from build123d import *

# Parameters (mm, degrees)
F0_W     = 20
F0_H     = 20
F1_DEPTH = 2
F2_W     = 20
F2_H     = 20
F3_DEPTH = 25
F5_W     = 9
F5_H     = 9
F6_DEPTH = 7
F7_R     = 1
F8_DEPTH = 18
F9_DEPTH = 24.8
F10_R    = 0.8
F11_R    = 0.8


with BuildPart() as f1:
    # F0 (on Top) → F1 (new body)
    with BuildSketch(Plane.XY):
        Rectangle(F0_W, F0_H)
    extrude(amount=F1_DEPTH)

    # F2 (on face) → F3 (join)
    with BuildSketch(Plane.XY.offset(2)):
        Rectangle(F2_W, F2_H)
        Polygon((0, -4.5), (-4.5, -4.5), (-4.5, 0), (-4.5, 4.5), (0, 4.5), (4.5, 4.5), (4.5, 0), (4.5, -4.5), align=None, mode=Mode.SUBTRACT)
    extrude(amount=F3_DEPTH)

    # F5 (on face) → F6 (cut)
    with BuildSketch(Plane.XY.offset(27)):
        Polygon((3.7816442632, -6.55), (7.5632885264, 0), (3.7816442632, 6.55), (-3.7816442632, 6.55), (-7.5632885264, 0), (-3.7816442632, -6.55), align=None)
        Rectangle(F5_W, F5_H, mode=Mode.SUBTRACT)
    extrude(amount=-F6_DEPTH, mode=Mode.SUBTRACT)

    # F7
    f7_edges = [f1.edges().sort_by_distance(p)[0] for p in [
        (3.781644, -6.55, 23.5),
        (7.563289, 0, 23.5),
        (3.781644, 6.55, 23.5),
        (-3.781644, 6.55, 23.5),
        (-7.563289, 0, 23.5),
        (-3.781644, -6.55, 23.5),
    ]]
    fillet(f7_edges, radius=F7_R)

    # F2 (on face) → F8 (join)
    with BuildSketch(Plane.XY.offset(2)):
        Rectangle(F2_W, F2_H)
        Polygon((0, -4.5), (-4.5, -4.5), (-4.5, 0), (-4.5, 4.5), (0, 4.5), (4.5, 4.5), (4.5, 0), (4.5, -4.5), align=None, mode=Mode.SUBTRACT)
        with BuildLine():
            ThreePointArc((4.5, 0), (3.1819805153, -3.1819805153), (0, -4.5))
            Line((0, -4.5), (4.5, -4.5))
            Line((4.5, -4.5), (4.5, 0))
        make_face()
        with BuildLine():
            Line((-4.5, 0), (-4.5, -4.5))
            Line((-4.5, -4.5), (0, -4.5))
            ThreePointArc((0, -4.5), (-3.1819805153, -3.1819805153), (-4.5, 0))
        make_face()
        with BuildLine():
            Line((-4.5, 4.5), (-4.5, 0))
            ThreePointArc((-4.5, 0), (-3.1819805153, 3.1819805153), (0, 4.5))
            Line((0, 4.5), (-4.5, 4.5))
        make_face()
        with BuildLine():
            ThreePointArc((0, 4.5), (3.1819805153, 3.1819805153), (4.5, 0))
            Line((4.5, 0), (4.5, 4.5))
            Line((4.5, 4.5), (0, 4.5))
        make_face()
    extrude(amount=F8_DEPTH)

    # F4 (on face) → F9 (cut, symmetric)
    with BuildSketch(Plane.XZ.offset(10)):
        with BuildLine():
            Line((-4.0082180343, 0), (4.0082180343, 0))
            ThreePointArc((4.0082180343, 0), (0, 4.0082180343), (-4.0082180343, 0))
        make_face()
    extrude(amount=F9_DEPTH, both=True, mode=Mode.SUBTRACT)

    # F10
    f10_edges = [f1.edges().sort_by_distance(p)[0] for p in [
        (4.008218, 0, 0),
        (-4.008218, 0, 0),
    ]]
    fillet(f10_edges, radius=F10_R)

    # F11
    f11_edges = [f1.edges().sort_by_distance(p)[0] for p in [
        (10, -10, 13.5),
        (-10, -10, 13.5),
        (-10, 10, 13.5),
        (10, 10, 13.5),
    ]]
    fillet(f11_edges, radius=F11_R)


solid = f1.part
Can you work these out from the model? Positions are in its coordinate system, mm. A direction names the side the tool comes from. Coordinates: 2 decimals unless noted, no trailing zeros. Write each loop counter-clockwise with the first axis right and the second up, starting at its lowest first coordinate (ties: lowest second). Pieces come first, ordered by that corner, then holes. Notation, with made-up numbers: (42.5, -24.75) - (51.5, -24.75) arc R13 cw to (51.5, -10.75) - close; hole circle Ø10 at (-27.5, -18.5). An arc over 180 degrees is marked (long way). Return JSON: item names as keys, results as strings. Group by question number.
Item 1: If we section it at C-C (y = 8.25): Write out the boundary of the cut face in (x, z), then the cut area to 3 significant figures.
Item 2: If we section it at A-A (z = 13): Write out the boundary of the cut face in (x, y), then the cut area to 3 significant figures.
Item 3: We'd pull the mould along X, two halves only. Please class faces 3 (the face through (4, 0, 2)), 4 (the face through (0, 7, 27)), 5 (the face through (10, 0, 13)): pulls with the +X half, pulls with the -X half, needs draft (parallel to the pull), parting line crosses it, or undercut.
Item 4: Which directions (+Z, -Z, +X, -X, +Y, -Y) give clear straight access to the entire face, cutting with the end or side of a thin tool? Please do faces 1 (the face through (9.76, 9.77, 13.31)), 2 (the face through (7.41, -0.01, 23.45)).
Item 5: If we section it at B-B (x = 1): Write out the boundary of the cut face in (y, z).
Item 6: If we section it at D-D (y = -4): Write out the boundary of the cut face in (x, z), then the cut area to 3 significant figures.
Item 7: Please list where these lines run through material, in increasing order: probe 1 along X at (y, z) = (-2, 15.5); probe 2 along X at (y, z) = (-1, 9); probe 3 along Y at (x, z) = (4, 20.75).
Item 8: I'm going to push flat-ended pins straight in: pin 1 Ø3 at (x, y) = (1.5, 0) entering from +Z; pin 2 Ø8 at (x, y) = (-2, 6.5) entering from -Z; pin 3 Ø4 at (x, y) = (3, -1) entering from +Z. Where does each tip first touch, or does it pass through?
Return value:
{
 "1": {"outline": "(-10, 0) - (-4.74, 0) arc R0.8 ccw to (-3.95, 0.67) arc R4.01 cw to (3.95, 0.67) arc R0.8 ccw to (4.74, 0) - (10, 0) - (10, 27) - (-10, 27) - close", "area": "515 mm^2"},
 "2": {"outline": "(-10, -9.2) arc R0.8 ccw to (-9.2, -10) - (9.2, -10) arc R0.8 ccw to (10, -9.2) - (10, 9.2) arc R0.8 ccw to (9.2, 10) - (-9.2, 10) arc R0.8 ccw to (-10, 9.2) - close; hole circle Ø9 at (0, 0)", "area": "336 mm^2"},
 "3": {"face 3": "undercut", "face 4": "needs draft", "face 5": "pulls with the +X half"},
 "4": {"face 1": "+Z, -Z, +X, +Y", "face 2": "+Z"},
 "5": {"outline": "(-10, 3.88) - (-4.39, 3.88) - (-4.39, 20) - (-6.55, 20) - (-6.55, 27) - (-10, 27) - close; (4.39, 3.88) - (10, 3.88) - (10, 27) - (6.55, 27) - (6.55, 20) - (4.39, 20) - close"},
 "6": {"outline": "(-10, 0) - (-4.74, 0) arc R0.8 ccw to (-3.95, 0.67) arc R4.01 cw to (-2.06, 3.44) - (-2.06, 20) - (-5.25, 20) - (-5.25, 27) - (-10, 27) - close; (2.06, 3.44) arc R4.01 cw to (3.95, 0.67) arc R0.8 ccw to (4.74, 0) - (10, 0) - (10, 27) - (5.25, 27) - (5.25, 20) - (2.06, 20) - close", "area": "374 mm^2"},
 "7": {"probe 1": "x = -10 to -4.03, 4.03 to 10", "probe 2": "x = -10 to -4.39, 4.39 to 10", "probe 3": "y = -10 to -6.16, 6.16 to 10"},
 "8": {"pin 1": "passes through", "pin 2": "stops at z = 0", "pin 3": "stops at z = 20"}
}
